```python
from build123d import *

# Parameters (mm, degrees)
F0_R     = 10.0651181203
F1_DEPTH = 25.4
F2_R     = 10.0651181203
F3_DEPTH = 25.4


with BuildPart() as f1:
    # F0 (on Top) → F1 (new body)
    with BuildSketch(Plane.XY):
        with BuildLine():
            Line((44.1251173615, 55.5551163852), (-62.9092976451, 55.5551163852))
            Line((-62.9092976451, 55.5551163852), (-62.9092976451, 42.5920749035))
            ThreePointArc((-62.9092976451, 42.5920749035), (-52.109599733, 50.8846190086), (-42.9095561607, 40.8467426896))
            ThreePointArc((-42.9095561607, 40.8467426896), (-52.109599733, 30.8088663707), (-62.9092976451, 39.1014104757))
            Line((-62.9092976451, 39.1014104757), (-62.9092976451, -2.5695350487))
            Line((-62.9092976451, -2.5695350487), (-61.6688355803, -2.5695350487))
            Line((-61.6688355803, -2.5695350487), (-61.6688355803, -8.0630239099))
            Line((-61.6688355803, -8.0630239099), (-62.9092976451, -8.0630239099))
            Line((-62.9092976451, -8.0630239099), (-62.9092976451, -54.3146505952))
            Line((-62.9092976451, -54.3146505952), (-55.1120936871, -54.3146505952))
            Line((-55.1120936871, -54.3146505952), (34.910235554, -54.3146505952))
            Line((34.910235554, -54.3146505952), (44.1251173615, -54.3146505952))
            Line((44.1251173615, -54.3146505952), (44.1251173615, 20.8220928907))
            Line((44.1251173615, 20.8220928907), (44.1251173615, 28.4420922399))
            Line((44.1251173615, 28.4420922399), (44.1251173615, 55.5551163852))
        make_face()
        Polygon((30.4799973965, -14.4425584003), (-45.1883710921, -18.3411631733), (26.7586056143, 15.8602334559), align=None, mode=Mode.SUBTRACT)
        with Locations((27.2902306169, 43.6820946634)):
            Circle(F0_R, mode=Mode.SUBTRACT)
    extrude(amount=F1_DEPTH)

    # F2 (on face) → F3 (join)
    with BuildSketch(Plane.XY.offset(25.4)):
        with BuildLine():
            ThreePointArc((-62.9092976451, 33.2274518748), (-37.8353474986, 26.1976296864), (-22.8169896281, 47.4713294781))
            ThreePointArc((-22.8169896281, 47.4713294781), (-23.1943629489, 51.5819332274), (-24.3138670359, 55.5551163852))
            Line((-24.3138670359, 55.5551163852), (-62.9092976451, 55.5551163852))
            Line((-62.9092976451, 55.5551163852), (-62.9092976451, 42.5920749035))
            ThreePointArc((-62.9092976451, 42.5920749035), (-42.9095561607, 40.8467426896), (-62.9092976451, 39.1014104757))
            Line((-62.9092976451, 39.1014104757), (-62.9092976451, 33.2274518748))
        make_face()
        with BuildLine():
            Line((39.7248882397, 55.5551163852), (17.9206636207, 55.5551163852))
            ThreePointArc((17.9206636207, 55.5551163852), (18.4737505401, 29.1833400362), (44.1251173615, 35.3301988385))
            Line((44.1251173615, 35.3301988385), (44.1251173615, 49.8539509685))
            ThreePointArc((44.1251173615, 49.8539509685), (42.2315107975, 52.9411002936), (39.7248882397, 55.5551163852))
        make_face()
        with Locations((27.2902306169, 43.6820946634)):
            Circle(F2_R, mode=Mode.SUBTRACT)
        with BuildLine():
            ThreePointArc((39.7248882397, 55.5551163852), (28.8227759302, 59.5300941875), (17.9206636207, 55.5551163852))
            Line((17.9206636207, 55.5551163852), (39.7248882397, 55.5551163852))
        make_face()
        with BuildLine():
            Line((44.1251173615, 49.8539509685), (44.1251173615, 35.3301988385))
            ThreePointArc((44.1251173615, 35.3301988385), (45.3468167725, 38.8701706187), (45.7607952142, 42.5920749035))
            ThreePointArc((45.7607952142, 42.5920749035), (45.3468167725, 46.3139791883), (44.1251173615, 49.8539509685))
        make_face()
    extrude(amount=F3_DEPTH)


solid = f1.part
```
Source: CAD feature listing. Evaluate the final solid. Frame: model axes, mm. A direction names the side the tool comes from. Coordinates: 2 decimals unless noted, no trailing zeros. Loops run counter-clockwise (first coordinate to the right, second up) from the corner with the lowest first, then second, coordinate; pieces in that order, holes last. Notation, with made-up numbers: M 80,-14.5 L 119,-14.5 A14 ccw 119,8.5 Z; hole C 86.5,31.25 d9. An arc over 180 degrees is marked long. Use a Markdown table: item, result. Add a question column.
Q1. Section query B-B, the plane x = -33.5. Return loops of the section in (y, z), and give its area (3 significant figures).
Q2. Draft query along Y for faces 1 (the flat face through (-21, 55.555, 19)), 2 (the flat face through (-61.669, -5, 13)), 3 (the flat face through (-10, -54.315, 13)), 4 (the flat face through (36, 35, 50.8)). Return one class per face: pulls with the +Y half, pulls with the -Y half, needs draft (parallel to the pull), parting line crosses it, or undercut.
Q3. Material intervals for L1, parallel to X at y = 40, z = 29; L2, parallel to Z at x = -57.5, y = -11; L3, parallel to Y at x = -9.5, z = 5, sorted ascending.
Q4. Access query for faces 5 (the flat face through (44.125, 0, 13)), 6 (the flat face through (43, 54, 25.4)), 7 (the flat face through (-6.825, -16.365, 12.522)), 8 (the flat face through (29, 57, 25.4)). Directions: +Z, -Z, +X, -X, +Y, -Y. A direction counts if a zero-diameter tool reaches every point of the face in a straight line with its end or side. Return the directions, or none.
Q5. Section query C-C, the plane x = 23. Return loops of the section in (y, z), and give its area (3 significant figures).
Q6. Section query D-D, the plane y = 3.5. Return loops of the section in (x, z).
Q7. Section query A-A, the plane z = 36.5. Return loops of the section in (x, y), and give its area (3 significant figures).
Q8. First-contact query: pin 1 (3 mm diameter, centred on x = -1.5, y = 40, fed in from +Z); pin 2 (1.6 mm diameter, centred on y = -4.5, z = 14, fed in from -X); pin 3 (3 mm diameter, centred on x = -25.5, z = 12.5, fed in from +Y); pin 4 (23 mm diameter, centred on x = 27.29, y = 43.68, fed in from -Z). Flat tips, straight axial feed; report the tip coordinate or a pass-through.
Result:
| question | item | result |
|---|---|---|
| 1 | outline | M -54.31,0 L -17.74,0 L -17.74,25.4 L -54.31,25.4 Z; M -12.78,0 L 55.56,0 L 55.56,50.8 L 28.28,50.8 L 28.28,25.4 L -12.78,25.4 Z |
| 1 | area | 3,360 mm2 |
| 2 | face 1 | pulls with the +Y half |
| 2 | face 2 | undercut |
| 2 | face 3 | pulls with the -Y half |
| 2 | face 4 | needs draft |
| 3 | L1 | x = -42.95 to -24.09, 12.08 to 17.92, 36.66 to 45.56 |
| 3 | L2 | z = 0 to 25.4 |
| 3 | L3 | y = -54.31 to -16.5, -1.38 to 55.56 |
| 4 | face 5 | -Z, +X, +Y, -Y |
| 4 | face 6 | +Z, +X, +Y |
| 4 | face 7 | +Z, -Z |
| 4 | face 8 | -Z, +X, -X, +Y |
| 5 | outline | M -54.31,0 L -14.83,0 L -14.83,25.4 L -54.31,25.4 Z; M 14.07,0 L 34.58,0 L 34.58,50.8 L 26.69,50.8 L 26.69,25.4 L 14.07,25.4 Z; M 52.79,0 L 55.56,0 L 55.56,25.4 L 58.5,25.4 L 58.5,50.8 L 52.79,50.8 Z |
| 5 | area | 1,940 mm2 |
| 6 | outline | M -62.91,0 L 0.76,0 L 0.76,25.4 L -62.91,25.4 Z; M 28.28,0 L 44.13,0 L 44.13,25.4 L 28.28,25.4 Z |
| 7 | outline | M -62.91,33.23 A22.58 ccw -24.31,55.56 L -62.91,55.56 L -62.91,42.59 A10.08 cw long -62.91,39.1 Z; C 28.82,42.59 d33.88; hole C 27.29,43.68 d20.13 |
| 7 | area | 1,340 mm2 |
| 8 | pin 1 | stops at z = 25.4 |
| 8 | pin 2 | stops at x = -61.67 |
| 8 | pin 3 | stops at y = 55.56 |
| 8 | pin 4 | stops at z = 0 |
